Here's how the part is built. I have some questions about the finished solid (model axes, mm). A direction names the side the tool comes from. Round coordinates to 2 decimals unless told otherwise and drop trailing zeros. Loops run counter-clockwise (first coordinate to the right, second up) from the corner with the lowest first, then second, coordinate; pieces in that order, holes last. Notation, with made-up numbers: (39, -2) - (53, -2) arc R18 cw to (53, 15) - close; hole circle Ø9 at (8, -31.75). An arc over 180 degrees is marked (long way). Answer as a JSON object with one key per item and string values. Group by question number.
1) I want a section at D-D, the plane x = -14. Please give me the cut outline in (y, z), then the cut area to 3 significant figures.
2) I want a section at C-C, the plane x = -2. Please give me the cut outline in (y, z), then the cut area to 3 significant figures.
3) I want a section at B-B, the plane z = -4.5. Please give me the cut outline in (x, y), then the cut area to 3 significant figures.
4) If we mould it in two halves opening along Z, with no side actions, what happens to faces 1 (the face through (20.248, 5.07, 17.287)), 2 (the face through (-12.3, -10, 4.3)), 3 (the face through (8, 2, 0))? For each: pulls with the +Z half, pulls with the -Z half, needs draft (parallel to the pull), parting line crosses it, or undercut.
5) Which directions (+Z, -Z, +X, -X, +Y, -Y) give clear straight access to the entire face, cutting with the end or side of a thin tool? Please do faces 4 (the face through (-7.5, 1, 0)), 5 (the face through (0, 0, -8)), 6 (the face through (0, 6, 11.5)).
6) If I drill on line 1 along X through (y, z) = (8.25, -8.5); line 2 along Z through (x, y) = (8, 4.5); line 3 along Z through (x, y) = (0, -2.5), over which ranges is the centre line in solid material (lowest first)? Write a range as [from, to].
7) I want a section at A-A, the plane y = 1. Please give me the cut outline in (x, z).
8) Will these pins go through, and if not, where does the flat tip stop? P1, Ø7.5, axis at x = -2, z = -5.5, coming from the -Y side; P2, Ø3, axis at y = -3, z = 12, coming from the -X side; P3, Ø1.5, axis at y = -1.5, z = 1, coming from the -X side.
from build123d import *

# Parameters (mm, degrees)
F0_W     = 42
F0_H     = 36
F1_DEPTH = 10
F2_R     = 18
F3_DEPTH = 10
F4_R     = 12.7
F5_DEPTH = 10
F6_W     = 23
F6_H     = 23
F7_DEPTH = 8
F8_W     = 15
F8_H     = 15
F9_DEPTH = 12.001
F10_R    = 1
F11_R    = 2.5


with BuildPart() as f1:
    # F0 (on Front) → F1 (new body)
    with BuildSketch(Plane.XZ):
        Rectangle(F0_W, F0_H)
    extrude(amount=-F1_DEPTH)

    # F2 (on Front) → F3 (join)
    with BuildSketch(Plane.XZ):
        Circle(F2_R)
    extrude(amount=F3_DEPTH)

    # F4 (on face) → F5 (cut)
    with BuildSketch(Plane.XZ.offset(10)):
        Circle(F4_R)
    extrude(amount=-F5_DEPTH, mode=Mode.SUBTRACT)

    # F6 (on face) → F7 (cut)
    with BuildSketch(Plane(origin=(0, 10, 0), x_dir=(-1, 0, 0), z_dir=(0, 1, 0))):
        Rectangle(F6_W, F6_H)
    extrude(amount=-F7_DEPTH, mode=Mode.SUBTRACT)

    # F8 (on face) → F9 (cut, through all)
    with BuildSketch(Plane(origin=(0, 2, 0), x_dir=(-1, 0, 0), z_dir=(0, 1, 0))):
        Rectangle(F8_W, F8_H)
    extrude(amount=-F9_DEPTH, mode=Mode.SUBTRACT)

    # F10
    f10_edges = [f1.edges().sort_by_distance(p)[0] for p in [
        (11.5, 6, 11.5),
        (-11.5, 6, 11.5),
        (11.5, 6, -11.5),
        (-11.5, 6, -11.5),
        (-7.5, 1, -7.5),
        (7.5, 1, -7.5),
        (7.5, 1, 7.5),
        (-7.5, 1, 7.5),
    ]]
    fillet(f10_edges, radius=F10_R)

    # F11
    f11_edges = [f1.edges().sort_by_distance(p)[0] for p in [
        (-21, 5, 18),
        (-21, 5, -18),
        (21, 5, 18),
        (21, 5, -18),
    ]]
    fillet(f11_edges, radius=F11_R)


solid = f1.part
Outcome:
{
 "1": {"outline": "(-10, -11.31) - (0, -11.31) - (0, -18) - (10, -18) - (10, 18) - (0, 18) - (0, 11.31) - (-10, 11.31) - close", "area": "586 mm^2"},
 "2": {"outline": "(-10, -17.89) - (0, -17.89) - (0, -18) - (10, -18) - (10, -11.5) - (2, -11.5) - (2, -7.5) - (0, -7.5) - (0, -12.54) - (-10, -12.54) - close; (-10, 12.54) - (0, 12.54) - (0, 7.5) - (2, 7.5) - (2, 11.5) - (10, 11.5) - (10, 18) - (0, 18) - (0, 17.89) - (-10, 17.89) - close", "area": "253 mm^2"},
 "3": {"outline": "(-21, 0) - (-17.43, 0) - (-17.43, -10) - (-11.88, -10) - (-11.88, 0) - (-7.5, 0) - (-7.5, 2) - (-11.5, 2) - (-11.5, 10) - (-21, 10) - close; (7.5, 0) - (11.88, 0) - (11.88, -10) - (17.43, -10) - (17.43, 0) - (21, 0) - (21, 10) - (11.5, 10) - (11.5, 2) - (7.5, 2) - close", "area": "317 mm^2"},
 "4": {"face 1": "pulls with the +Z half", "face 2": "needs draft", "face 3": "undercut"},
 "5": {"face 4": "+Y, -Y", "face 5": "-Y", "face 6": "+Y"},
 "6": {"line 1": "[-21, -11.5], [11.5, 21]", "line 2": "[-18, -11.5], [11.5, 18]", "line 3": "[-18, -12.7], [12.7, 18]"},
 "7": {"outline": "(-21, -15.5) arc R2.5 ccw to (-18.5, -18) - (18.5, -18) arc R2.5 ccw to (21, -15.5) - (21, 15.5) arc R2.5 ccw to (18.5, 18) - (-18.5, 18) arc R2.5 ccw to (-21, 15.5) - close; hole (-7.5, -6.5) arc R1 ccw to (-6.5, -7.5) - (6.5, -7.5) arc R1 ccw to (7.5, -6.5) - (7.5, 6.5) arc R1 ccw to (6.5, 7.5) - (-6.5, 7.5) arc R1 ccw to (-7.5, 6.5) - close"},
 "8": {"P1": "y = 0", "P2": "x = -14.62", "P3": "x = -18"}
}
